Check sheet for the modelled part. Datum: model origin and axes. Units: mm. Give positions to 0.01 mm unless a question says otherwise; leave off trailing zeros. Loops run counter-clockwise (first coordinate to the right, second up) from the corner with the lowest first, then second, coordinate; pieces in that order, holes last. Notation, with made-up numbers: M 54,31 L 108,31 A16 ccw 108,49 Z; hole C 73.25,2 d3. An arc over 180 degrees is marked long. Use one line per item in the form item = value.
from build123d import *

# Parameters (mm, degrees)
F1_DEPTH  = 30.6234291007
F13_DEPTH = 50
F14_DEPTH = 500
F15_DEPTH = 500
F16_DEPTH = 500
F17_DEPTH = 500
F24_DEPTH = 500
F25_DEPTH = 500
F26_DEPTH = 500
F27_DEPTH = 500
F28_DEPTH = 500


with BuildPart() as f1:
    # F0 (on Top) → F1 (new body, symmetric)
    with BuildSketch(Plane.XY):
        Polygon((-36, 11.6971090644), (-36, -11.6971090644), (-22.249223595, -30.6234291007), (0, -37.8526400726), (22.249223595, -30.6234291007), (36, -11.6971090644), (36, 11.6971090644), (22.249223595, 30.6234291007), (0, 37.8526400726), (-22.249223595, 30.6234291007), align=None)
    extrude(amount=F1_DEPTH, both=True)

    # F3 (on Right) → F13 (cut, symmetric)
    with BuildSketch(Plane.YZ):
        Polygon((-37.8526400726, -7.2292109719), (-18.9263200363, 30.6234291007), (-37.8526400726, 30.6234291007), align=None)
    extrude(amount=F13_DEPTH, both=True, mode=Mode.SUBTRACT)

    # F6 (on face) → F14 (cut, symmetric)
    with BuildSketch(Plane(origin=(0, 0, 0), x_dir=(-0.9510565163, 0.3090169944, 0), z_dir=(0.3090169944, 0.9510565163, 0))):
        Polygon((-37.8526400726, -7.2292109719), (-18.9263200363, 30.6234291007), (-37.8526400726, 30.6234291007), align=None)
    extrude(amount=F14_DEPTH, both=True, mode=Mode.SUBTRACT)

    # F8 (on face) → F15 (cut, symmetric)
    with BuildSketch(Plane(origin=(0, 0, 0), x_dir=(0.5877852523, 0.8090169944, 0), z_dir=(0.8090169944, -0.5877852523, 0))):
        Polygon((37.8526400726, -7.2292109719), (37.8526400726, 30.6234291007), (18.9263200363, 30.6234291007), align=None)
    extrude(amount=F15_DEPTH, both=True, mode=Mode.SUBTRACT)

    # F10 (on face) → F16 (cut, symmetric)
    with BuildSketch(Plane(origin=(0, 0, 0), x_dir=(0.5877852523, -0.8090169944, 0), z_dir=(-0.8090169944, -0.5877852523, 0))):
        Polygon((-18.9263200363, 30.6234291007), (-37.8526400726, 30.6234291007), (-37.8526400726, -7.2292109719), align=None)
    extrude(amount=F16_DEPTH, both=True, mode=Mode.SUBTRACT)

    # F12 (on face) → F17 (cut, symmetric)
    with BuildSketch(Plane(origin=(0, 0, 0), x_dir=(-0.9510565163, -0.3090169944, 0), z_dir=(-0.3090169944, 0.9510565163, 0))):
        Polygon((37.8526400726, 26.069773404), (37.8526400726, 30.6234291007), (18.9263200363, 30.6234291007), (37.8526400726, -7.2292109719), align=None)
    extrude(amount=F17_DEPTH, both=True, mode=Mode.SUBTRACT)

    # F19 (on Right) → F24 (cut, symmetric)
    with BuildSketch(Plane.YZ):
        Polygon((37.8526400726, 7.2292109719), (18.9263200363, -30.6234291007), (37.8526400726, -30.6234291007), align=None)
    extrude(amount=F24_DEPTH, both=True, mode=Mode.SUBTRACT)

    # F20 (on face) → F25 (cut, symmetric)
    with BuildSketch(Plane(origin=(0, 0, 0), x_dir=(-0.9510565163, -0.3090169944, 0), z_dir=(-0.3090169944, 0.9510565163, 0))):
        Polygon((-37.8526400726, -30.6234291007), (-18.9263200363, -30.6234291007), (-37.8526400726, 7.2292109719), align=None)
    extrude(amount=F25_DEPTH, both=True, mode=Mode.SUBTRACT)

    # F21 (on face) → F26 (cut, symmetric)
    with BuildSketch(Plane(origin=(0, 0, 0), x_dir=(0.5877852523, -0.8090169944, 0), z_dir=(-0.8090169944, -0.5877852523, 0))):
        Polygon((37.8526400726, 7.2292109719), (18.9263200363, -30.6234291007), (37.8526400726, -30.6234291007), align=None)
    extrude(amount=F26_DEPTH, both=True, mode=Mode.SUBTRACT)

    # F22 (on face) → F27 (cut, symmetric)
    with BuildSketch(Plane(origin=(0, 0, 0), x_dir=(0.5877852523, 0.8090169944, 0), z_dir=(0.8090169944, -0.5877852523, 0))):
        Polygon((-37.8526400726, -30.6234291007), (-18.9263200363, -30.6234291007), (-37.8526400726, 7.2292109719), align=None)
    extrude(amount=F27_DEPTH, both=True, mode=Mode.SUBTRACT)

    # F23 (on face) → F28 (cut, symmetric)
    with BuildSketch(Plane(origin=(0, 0, 0), x_dir=(-0.9510565163, 0.3090169944, 0), z_dir=(0.3090169944, 0.9510565163, 0))):
        Polygon((37.8526400726, 7.2292109719), (18.9263200363, -30.6234291007), (37.8526400726, -30.6234291007), align=None)
    extrude(amount=F28_DEPTH, both=True, mode=Mode.SUBTRACT)


solid = f1.part
1) Section check D-D (y = -25). Record the cut outline in (x, z), then the cut area to 3 significant figures.
Evaluation:
outline = M -26.33,2.93 L 0,-28.03 L 26.33,2.93 L 18.16,18.48 L -18.16,18.48 Z
area = 1,510 mm^2
2) Section check C-C (y = -15.5). Record the cut outline in (x, z).
Evaluation:
outline = M -33.24,-4.32 L -10.87,-30.62 L 10.87,-30.62 L 33.24,-4.32 L 14.86,30.62 L -14.86,30.62 Z
3) Release check for a two-part mould opening along Y. For faces 1 (the face through (0, -2, 30.623)), 2 (the face through (26.78, 9.03, -11.96)), 3 (the face through (-16.36, -23.04, -11.96)) record: pulls with the +Y half, pulls with the -Y half, needs draft (parallel to the pull), parting line crosses it, or undercut.
Evaluation:
face_1 = needs draft
face_2 = pulls with the +Y half
face_3 = pulls with the -Y half
4) Scan lines: line 1 (Z direction, x = -6, y = -26); line 2 (X direction, y = -28, z = -3.5); line 3 (Z direction, x = -27, y = -16). Record each from-to range of solid material in increasing order.
Evaluation:
line_1 = -19.35 to 16.48
line_2 = -16.73 to 16.73
line_3 = -10.85 to 7.23
5) Section check A-A (x = -20). Record the cut outline in (y, z), then the cut area to 3 significant figures.
Evaluation:
outline = M -31.35,5.77 L -8.86,-30.62 L -0.31,-30.62 L 27.53,-13.42 L 31.35,-5.77 L 8.86,30.62 L 0.31,30.62 L -27.53,13.42 Z
area = 2,380 mm^2
6) Section check B-B (z = -5). Record the cut outline in (x, y), then the cut area to 3 significant figures.
Evaluation:
outline = M -36,-8.09 L -33.88,-14.62 L -3.43,-36.74 L 3.43,-36.74 L 33.88,-14.62 L 36,-8.09 L 24.37,27.71 L 18.82,31.74 L -18.82,31.74 L -24.37,27.71 Z
area = 3,620 mm^2
7) Depth check by flat-ended pin: pin 1 Ø1.5 at (y, z) = (-20.5, -13.5) entering from +X; pin 2 Ø6 at (y, z) = (-2, 12.5) entering from -X; pin 3 Ø4 at (x, z) = (19, 1.5) entering from +Y. Enter the tip coordinate at first touch or a pass-through.
Evaluation:
pin_1 = 19.76
pin_2 = -30.63
pin_3 = 29.5
